```python
from build123d import *

# Parameters (mm, degrees)
SKETCH_1_R                  = 4.5
SKETCH_1_R_2                = 1.6
EXTRUDE_1_DEPTH             = 3
SKETCH_2_R                  = 1.6
EXTRUDE_2_DEPTH             = 2
EXTRUDE_3_DEPTH             = 24
CUT_EXTRUDE_1_REACH         = 88.596
SKETCH_4_R                  = 1.6
SKETCH_6_W                  = 9
SKETCH_6_H                  = 13.66994387
CUT_EXTRUDE_2_DEPTH         = 3
CUT_EXTRUDE_3_REACH         = 88.648
SKETCH_7_R                  = 3
EXTRUDE_START               = 3
SKETCH_8_R                  = 4.5
SKETCH_8_R_2                = 1.6
EXTRUDE_4_DEPTH             = 3
CUT_EXTRUDE_4_REACH         = 88.596
SKETCH_9_R                  = 6
SKETCH_10_W                 = 51
SKETCH_10_H                 = 0.8
EXTRUDE_5_DEPTH             = 2
SKETCH_11_W                 = 81.2
SKETCH_11_H                 = 2
EXTRUDE_6_DEPTH             = 1
EXTRUDE_6_DIRECTION_2_REACH = 88.227
FILLET_1_R                  = 10
CUT_EXTRUDE_5_REACH         = 88.355
SKETCH_12_W                 = 45
SKETCH_12_H                 = 0.8
EXTRUDE_7_DEPTH             = 24
EXTRUDE_8_DEPTH             = 9
CUT_EXTRUDE_START           = -2.144737
SKETCH_15_W                 = 21.643481228
SKETCH_15_H                 = 2
CUT_EXTRUDE_6_DEPTH         = 2.144737
CUT_EXTRUDE_7_REACH         = 88.157


with BuildPart() as part:
    # 草图1 → 凸台-拉伸1 (new body)
    with BuildSketch(Plane(origin=(0, 0, 0), x_dir=(1, 0, 0), z_dir=(0, 1, 0))):
        with Locations(Location((0, 0, 0), (0, 0, 270))):
            Circle(SKETCH_1_R)
        with Locations(Location((0, 0, 0), (0, 0, 270))):
            Circle(SKETCH_1_R_2, mode=Mode.SUBTRACT)
    extrude(amount=EXTRUDE_1_DEPTH)

    # 草图2 → 凸台-拉伸2 (add)
    with BuildSketch(Plane(origin=(0, 3, 0), x_dir=(1, 0, 0), z_dir=(0, 1, 0))):
        with BuildLine():
            Line((0, 4.5), (81.2, 4.5))
            ThreePointArc((81.2, 4.5), (85.7, 0), (81.2, -4.5))
            Line((81.2, -4.5), (0, -4.5))
            ThreePointArc((0, -4.5), (-4.5, 0), (0, 4.5))
        make_face()
        with Locations(Location((81.2, 0, 0), (0, 0, 270))):
            Circle(SKETCH_2_R, mode=Mode.SUBTRACT)
        with Locations(Location((0, 0, 0), (0, 0, 270))):
            Circle(SKETCH_2_R, mode=Mode.SUBTRACT)
    extrude(amount=EXTRUDE_2_DEPTH)

    # 草图3 → 凸台-拉伸3 (add)
    with BuildSketch(Plane(origin=(75, 0, 0), x_dir=(0, 0, -1), z_dir=(1, 0, 0))):
        Polygon((-4.5, 5), (4.5, 13.392635775), (4.5, 5), align=None)
    extrude(amount=-EXTRUDE_3_DEPTH)

    # 草图4 → 切除-拉伸1 (cut, up to next)
    with BuildSketch(Plane(origin=(0, 4.918910297, 4.58695806), x_dir=(1, 0, 0), z_dir=(0, 0.7313537016191739, 0.6819983600624948)), mode=Mode.PRIVATE) as cut_extrude_1_sk1:
        with Locations(Location((54.5, 6.271873718, 0), (0, 0, 270))):
            Circle(SKETCH_4_R)
    cut_extrude_1_tool1 = extrude(cut_extrude_1_sk1.sketch, amount=-CUT_EXTRUDE_1_REACH, mode=Mode.PRIVATE) & part.part
    # 草图4 → 切除-拉伸1 (cut, up to next)
    with BuildSketch(Plane(origin=(0, 4.918910297, 4.58695806), x_dir=(1, 0, 0), z_dir=(0, 0.7313537016191739, 0.6819983600624948)), mode=Mode.PRIVATE) as cut_extrude_1_sk2:
        with Locations(Location((71.5, 6.271873718, 0), (0, 0, 270))):
            Circle(SKETCH_4_R)
    cut_extrude_1_tool2 = extrude(cut_extrude_1_sk2.sketch, amount=-CUT_EXTRUDE_1_REACH, mode=Mode.PRIVATE) & part.part
    add(cut_extrude_1_tool1.solids().sort_by_distance((54.5, 9.196318, 0))[0], mode=Mode.SUBTRACT)
    add(cut_extrude_1_tool2.solids().sort_by_distance((71.5, 9.196318, 0))[0], mode=Mode.SUBTRACT)

    # 草图6 → 切除-拉伸2 (cut)
    with BuildSketch(Plane(origin=(0, 4.918910297, 4.58695806), x_dir=(1, 0, 0), z_dir=(0, 0.7313537016191739, 0.6819983600624948))):
        with Locations((63, 5.589875358)):
            Rectangle(SKETCH_6_W, SKETCH_6_H)
    extrude(amount=-CUT_EXTRUDE_2_DEPTH, mode=Mode.SUBTRACT)

    # 草图7 → 切除-拉伸3 (cut, up to next)
    with BuildSketch(Plane(origin=(0, 2.724849193, 2.54096298), x_dir=(1, 0, 0), z_dir=(0, 0.7313537016191739, 0.6819983600624948)), mode=Mode.PRIVATE) as cut_extrude_3_sk1:
        with Locations(Location((54.5, 6.271873718, 0), (0, 0, 270))):
            Circle(SKETCH_7_R)
    cut_extrude_3_tool1 = extrude(cut_extrude_3_sk1.sketch, amount=-CUT_EXTRUDE_3_REACH, mode=Mode.PRIVATE) & part.part
    # 草图7 → 切除-拉伸3 (cut, up to next)
    with BuildSketch(Plane(origin=(0, 2.724849193, 2.54096298), x_dir=(1, 0, 0), z_dir=(0, 0.7313537016191739, 0.6819983600624948)), mode=Mode.PRIVATE) as cut_extrude_3_sk2:
        with Locations(Location((71.5, 6.271873718, 0), (0, 0, 270))):
            Circle(SKETCH_7_R)
    cut_extrude_3_tool2 = extrude(cut_extrude_3_sk2.sketch, amount=-CUT_EXTRUDE_3_REACH, mode=Mode.PRIVATE) & part.part
    add(cut_extrude_3_tool1.solids().sort_by_distance((54.5, 7.002257, -2.045995))[0], mode=Mode.SUBTRACT)
    add(cut_extrude_3_tool2.solids().sort_by_distance((71.5, 7.002257, -2.045995))[0], mode=Mode.SUBTRACT)

    # 草图8 → 凸台-拉伸4 (add)
    with BuildSketch(Plane.XZ.offset(-3).offset(EXTRUDE_START)):
        with Locations(Location((81.2, 0, 0), (0, 0, 90))):
            Circle(SKETCH_8_R)
        with Locations(Location((81.2, 0, 0), (0, 0, 90))):
            Circle(SKETCH_8_R_2, mode=Mode.SUBTRACT)
    extrude(amount=-EXTRUDE_4_DEPTH)

    # 草图9 → 切除-拉伸4 (cut, up to next)
    with BuildSketch(Plane(origin=(0, 4.918910297, 4.58695806), x_dir=(1, 0, 0), z_dir=(0, 0.7313537016191739, 0.6819983600624948)), mode=Mode.PRIVATE) as cut_extrude_4_sk1:
        with Locations((77.925, 13.271873718)):
            Circle(SKETCH_9_R)
    cut_extrude_4_tool1 = extrude(cut_extrude_4_sk1.sketch, amount=-CUT_EXTRUDE_4_REACH, mode=Mode.PRIVATE) & part.part
    add(cut_extrude_4_tool1.solids().sort_by_distance((77.925, 13.970306, -5.119476))[0], mode=Mode.SUBTRACT)

    # 草图10 → 凸台-拉伸5 (add)
    with BuildSketch(Plane(origin=(0, 5, 0), x_dir=(1, 0, 0), z_dir=(0, 1, 0))):
        with Locations((25.5, 4.1)):
            Rectangle(SKETCH_10_W, SKETCH_10_H)
    extrude(amount=EXTRUDE_5_DEPTH)

    # 草图11 → 凸台-拉伸6 (add)
    with BuildSketch(Plane(origin=(0, 5, 0), x_dir=(1, 0, 0), z_dir=(0, 1, 0))):
        with Locations((40.6, -5.5)):
            Rectangle(SKETCH_11_W, SKETCH_11_H)
    extrude(amount=EXTRUDE_6_DEPTH)

    # 凸台-拉伸6 direction 2: up to this face of the body (flat: up to its plane)
    extrude_6_direction_2_end = Plane(part.part.faces().sort_by_distance((39.023781637, 3, 0.016114568))[0])
    # 草图11 → 凸台-拉伸6 direction 2 (add, up to the picked face)
    with BuildSketch(Plane(origin=(0, 5, 0), x_dir=(1, 0, 0), z_dir=(0, 1, 0)), mode=Mode.PRIVATE) as extrude_6_direction_2_sk1:
        with Locations((40.6, -5.5)):
            Rectangle(SKETCH_11_W, SKETCH_11_H)
    extrude_6_direction_2_tool1 = split(extrude(extrude_6_direction_2_sk1.sketch, amount=-EXTRUDE_6_DIRECTION_2_REACH, mode=Mode.PRIVATE), bisect_by=extrude_6_direction_2_end, keep=Keep.BOTH, mode=Mode.PRIVATE)
    add(extrude_6_direction_2_tool1.solids().sort_by(Axis((40.6, 5, 5.5), (0, -1, 0)))[0])

    # 圆角1
    # the kernel refuses this fillet: 10 mm, written as the material it adds along each edge
    with BuildSketch(Plane(origin=(81.2, 3, 4.5), x_dir=(0.9510569298520609, 0, -0.30901572157476376), z_dir=(0, 1, 0))) as fillet_1_piece_1:
        with BuildLine():
            CenterArc((5.87129871, -9.510569299), FILLET_1_R, 107.999923321, 22.461280704)
            Line((-0.618031443, -1.90211386), (0, 0))
            ThreePointArc((0, 0), (1.390570747, -0.220243816), (2.781141494, 0))
        make_face()
    extrude(amount=2)
    with BuildSketch(Plane(origin=(0, 3, 4.5), x_dir=(-0.9510569298520611, 0, -0.3090157215747629), z_dir=(0, 1, 0))) as fillet_1_piece_2:
        with BuildLine():
            CenterArc((5.87129871, 9.510569299), FILLET_1_R, 229.538795975, 22.461280704)
            Line((-0.618031443, 1.90211386), (0, 0))
            ThreePointArc((0, 0), (1.390570747, 0.220243816), (2.781141494, 0))
        make_face()
    extrude(amount=2)

    # 草图12 → 切除-拉伸5 (cut, up to next)
    with BuildSketch(Plane(origin=(0, 5, 0), x_dir=(1, 0, 0), z_dir=(0, 1, 0)), mode=Mode.PRIVATE) as cut_extrude_5_sk1:
        with Locations((28.5, -4.9)):
            Rectangle(SKETCH_12_W, SKETCH_12_H)
    cut_extrude_5_tool1 = extrude(cut_extrude_5_sk1.sketch, amount=CUT_EXTRUDE_5_REACH, mode=Mode.PRIVATE) & part.part
    add(cut_extrude_5_tool1.solids().sort_by_distance((28.5, 5, 4.9))[0], mode=Mode.SUBTRACT)

    # 草图13 → 凸台-拉伸7 (add)
    with BuildSketch(Plane(origin=(75, 0, 0), x_dir=(0, 0, -1), z_dir=(1, 0, 0))):
        Polygon((-4.5, 6), (-3.42763129, 6), (-4.5, 5), align=None)
    extrude(amount=-EXTRUDE_7_DEPTH)

    # 草图14 → 凸台-拉伸8 (add)
    with BuildSketch(Plane(origin=(58.5, 0, 0), x_dir=(0, 0, -1), z_dir=(1, 0, 0))):
        Polygon((-3.42763129, 6), (-1.38163621, 3.805938895), (-2.245899863, 3), (-4.5, 3), (-4.5, 5), align=None)
    extrude(amount=EXTRUDE_8_DEPTH)

    # 草图15 → 切除-拉伸6 (cut)
    with BuildSketch(Plane(origin=(0, 4.918910297, 4.58695806), x_dir=(1, 0, 0), z_dir=(0, 0.7313537016191739, 0.6819983600624948)).offset(CUT_EXTRUDE_START)):
        with Locations((61.821740614, 11.424847293)):
            Rectangle(SKETCH_15_W, SKETCH_15_H)
    extrude(amount=CUT_EXTRUDE_6_DEPTH, mode=Mode.SUBTRACT)

    # 草图16 → 切除-拉伸7 (cut, up to next)
    with BuildSketch(Plane(origin=(0, 6, 0), x_dir=(1, 0, 0), z_dir=(0, 1, 0)), mode=Mode.PRIVATE) as cut_extrude_7_sk1:
        with BuildLine():
            Line((79.900166375, -6.5), (81.2, -6.5))
            ThreePointArc((81.2, -6.5), (81.518478449, -6.013408883), (81.864704052, -5.546153846))
            ThreePointArc((81.864704052, -5.546153846), (80.992094803, -6.24893137), (79.900166375, -6.5))
        make_face()
    cut_extrude_7_tool1 = extrude(cut_extrude_7_sk1.sketch, amount=-CUT_EXTRUDE_7_REACH, mode=Mode.PRIVATE) & part.part
    add(cut_extrude_7_tool1.solids().sort_by_distance((81.054691, 6, 6.297183))[0], mode=Mode.SUBTRACT)


solid = part.part
```
Input: part model. Units: mm. Frame: model coordinates. A direction names the side the tool comes from. Give positions to 0.01 mm unless a question says otherwise; leave off trailing zeros. Order: outer loops, then holes, each group sorted by start corner. A loop starts at its lowest first (then second) coordinate and runs counter-clockwise, first axis right, second up. Notation, with made-up numbers: (-39.75, -14.75) -> (-33.75, -14.75) arc R9 cw to (-33.75, -9.75) -> close; hole circle Ø11 at (73.5, -4). An arc over 180 degrees is marked (long way). Write each question's results on one line, items separated by ' | '. Start each with the question number.
Item 1: Contact query for flat-ended pins moving along their axis: P1, Ø3, axis at x = 79.5, z = 2, coming from the +Y side; P2, Ø6, axis at x = 65.5, z = -0.5, coming from the -Y side; P3, Ø3.5, axis at x = 24, z = 5.5, coming from the +Y side. Output: stop coordinate, or through.
Item 2: Cut plane C-C on z = 2.5. Return the cut outline in (x, y), then the cut area to 3 significant figures.
Item 3: Cut plane D-D on x = 62.5. Return the cut outline in (y, z).
Item 4: Line query: line 1 (X direction, y = 3.7, z = 0); line 2 (X direction, y = 2.85, z = 0); line 3 (Z direction, x = 81.2, y = 3.7). Output: solid intervals per line, ascending.
Item 5: Cut plane B-B on x = 38.5. Return the cut outline in (y, z).
Item 6: Mould query, pull axis Z, two halves, no side actions, for faces 1 (the cylindrical face through (73.086, 8.257, -1.161)), 2 (the flat face through (41, 3, 1)), 3 (the flat face through (69.64, 8.97, 0.24)). Classes: pulls with the +Z half, pulls with the -Z half, needs draft (parallel to the pull), parting line crosses it, or undercut.
Item 7: Set-up query: faces 4 (the flat face through (39, 5, 6.5)), 5 (the flat face through (58.5, 8, -1)), 6 (the flat face through (41, 6, 6)), 7 (the flat face through (75, 7, -1)), 8 (the cylindrical face through (53.351, 3.827, -1.217)). Return all of +Z, -Z, +X, -X, +Y, -Y with unobstructed straight access to the full face (end or side cutting, diameter ignored); none if empty.
Item 8: Cut plane A-A on y = 1. Return the cut outline in (x, z), then the cut area to 3 significant figures.
Established:
1) P1: y = 5 | P2: y = 3 | P3: y = 6
2) outline: (-3.74, 0) -> (3.74, 0) -> (3.74, 3) -> (77.46, 3) -> (77.46, 0) -> (84.94, 0) -> (84.94, 5) -> (75, 5) -> (75, 6.87) -> (67.5, 6.87) -> (67.5, 5.01) -> (58.5, 5.01) -> (58.5, 6.87) -> (51, 6.87) -> (51, 5) -> (-3.74, 5) -> close | area: 250 mm^2
3) outline: (3, -4.5) -> (9.29, -4.5) -> (3.81, 1.38) -> (6, 3.43) -> (6, 6.5) -> (3, 6.5) -> close
4) line 1: -4.5 to -1.6, 1.6 to 79.6, 82.8 to 85.7 | line 2: -4.5 to -1.6, 1.6 to 4.5, 76.7 to 79.6, 82.8 to 85.7 | line 3: -4.5 to -1.6, 1.6 to 6.14
5) outline: (3, -4.5) -> (7, -4.5) -> (7, -3.7) -> (5, -3.7) -> (5, 5.3) -> (6, 5.3) -> (6, 6.5) -> (3, 6.5) -> close
6) face 1: undercut | face 2: needs draft | face 3: pulls with the +Z half
7) face 4: +Z, +X, -X, +Y, -Y | face 5: +Y | face 6: +Z, +X, -X, +Y | face 7: -Z, +X, +Y | face 8: none
8) outline: circle Ø9 at (0, 0); circle Ø9 at (81.2, 0); hole circle Ø3.2 at (0, 0); hole circle Ø3.2 at (81.2, 0) | area: 111 mm^2
